from build123d import *

# Parameters (mm, degrees)
SKETCH1_R           = 4.05
BOSS_EXTRUDE1_DEPTH = 40
SKETCH2_R           = 2.75
CUT_EXTRUDE1_DEPTH  = 40
CHAMFER1_SIZE       = 5
SKETCH4_W           = 15
SKETCH4_H           = 40
BOSS_EXTRUDE2_DEPTH = 20
SKETCH5_R           = 2.75
BOSS_EXTRUDE3_DEPTH = 3
CHAMFER2_SIZE       = 5
CHAMFER3_SIZE       = 5
BOSS_EXTRUDE4_START = -5
SKETCH6_R           = 4.05
BOSS_EXTRUDE4_DEPTH = 5
SKETCH7_R           = 1.95
CUT_EXTRUDE2_DEPTH  = 20
CHAMFER4_SIZE       = 2
CHAMFER5_SIZE       = 3
SKETCH8_R           = 3
SKETCH8_R_2         = 2.75
BOSS_EXTRUDE5_DEPTH = 0.5
CHAMFER6_SIZE       = 0.5
BOSS_EXTRUDE6_START = 0.5
SKETCH9_R           = 3
SKETCH9_R_2         = 2.75
BOSS_EXTRUDE6_DEPTH = 0.5
CHAMFER7_SIZE       = 0.5


with BuildPart() as part:
    # Sketch1 → Boss-Extrude1 (new body)
    with BuildSketch(Plane.XY):
        Polygon((-20.25, 0), (20.25, 0), (20.25, -27), (41.75, -27), (41.75, 7), (-41.75, 7), (-41.75, -27), (-20.25, -27), align=None)
        with Locations((31.75, -10)):
            Circle(SKETCH1_R, mode=Mode.SUBTRACT)
        with Locations(Location((-31.75, -10, 0), (0, 0, 180))):
            Circle(SKETCH1_R, mode=Mode.SUBTRACT)
    extrude(amount=BOSS_EXTRUDE1_DEPTH)

    # Sketch2 → Cut-Extrude1 (cut)
    with BuildSketch(Plane(origin=(0, 0, 0), x_dir=(-1, 0, 0), z_dir=(0, -1, 0))):
        with Locations(Location((0, -30, 0), (0, 0, 90))):
            Circle(SKETCH2_R)
    extrude(amount=-CUT_EXTRUDE1_DEPTH, mode=Mode.SUBTRACT)

    # Chamfer1
    chamfer1_edges = [part.edges().sort_by_distance(p)[0] for p in [
        (41.75, 7, 20),
    ]]
    chamfer(chamfer1_edges, length=CHAMFER1_SIZE)

    # Sketch4 → Boss-Extrude2 (add)
    with BuildSketch(Plane(origin=(0, 7, 0), x_dir=(1, 0, 0), z_dir=(0, 1, 0))):
        with Locations((29.25, -20)):
            Rectangle(SKETCH4_W, SKETCH4_H)
    extrude(amount=BOSS_EXTRUDE2_DEPTH)

    # Sketch5 → Boss-Extrude3 (add)
    with BuildSketch(Plane(origin=(0, 27, 0), x_dir=(1, 0, 0), z_dir=(0, 1, 0))):
        with BuildLine():
            Line((20.579588566, -40), (21.75, -40))
            Line((21.75, -40), (36.75, -40))
            Line((36.75, -40), (36.75, 0))
            Line((36.75, 0), (21.75, 0))
            Line((21.75, 0), (-4.223300645, -25.738107033))
            ThreePointArc((-4.223300645, -25.738107033), (-5.538041345, -27.691299485), (-6, -30))
            Line((-6, -30), (-6, -40))
            Line((-6, -40), (20.579588566, -40))
        make_face()
        with Locations(Location((0, -30, 0), (0, 0, 90))):
            Circle(SKETCH5_R, mode=Mode.SUBTRACT)
    extrude(amount=BOSS_EXTRUDE3_DEPTH)

    # Chamfer2
    chamfer2_edges = [part.edges().sort_by_distance(p)[0] for p in [
        (36.75, 30, 20),
    ]]
    chamfer(chamfer2_edges, length=CHAMFER2_SIZE)

    # Chamfer3
    chamfer3_edges = [part.edges().sort_by_distance(p)[0] for p in [
        (-41.75, 7, 20),
    ]]
    chamfer(chamfer3_edges, length=CHAMFER3_SIZE)

    # Sketch6 → Boss-Extrude4 (add)
    with BuildSketch(Plane.XY.offset(40).offset(BOSS_EXTRUDE4_START)):
        with Locations(Location((-31.75, -10, 0), (0, 0, 180))):
            Circle(SKETCH6_R)
        with Locations((31.75, -10)):
            Circle(SKETCH6_R)
    extrude(amount=BOSS_EXTRUDE4_DEPTH)

    # Sketch7 → Cut-Extrude2 (cut)
    with BuildSketch(Plane(origin=(0, -27, 0), x_dir=(-1, 0, 0), z_dir=(0, -1, 0))):
        with Locations(Location((-31, -5, 0), (0, 0, 90))):
            Circle(SKETCH7_R)
        with Locations(Location((-31, -25, 0), (0, 0, 90))):
            Circle(SKETCH7_R)
    cut_extrude2 = extrude(amount=-CUT_EXTRUDE2_DEPTH, mode=Mode.SUBTRACT)

    # Mirror1: Cut-Extrude2 across plane
    add(cut_extrude2.mirror(Plane(origin=(0, 0, 0), x_dir=(0, 0, 1), z_dir=(1, 0, 0))), mode=Mode.SUBTRACT)

    # Chamfer4
    chamfer4_edges = [part.edges().sort_by_distance(p)[0] for p in [
        (-6, 28.5, 40),
    ]]
    chamfer(chamfer4_edges, length=CHAMFER4_SIZE)

    # Chamfer5
    chamfer5_edges = [part.edges().sort_by_distance(p)[0] for p in [
        (21.75, 7, 20),
        (21.75, 27, 20),
    ]]
    chamfer(chamfer5_edges, length=CHAMFER5_SIZE)

    # Sketch8 → Boss-Extrude5 (add)
    with BuildSketch(Plane(origin=(0, 7, 0), x_dir=(1, 0, 0), z_dir=(0, 1, 0))):
        with Locations(Location((0, -30, 0), (0, 0, 90))):
            Circle(SKETCH8_R)
        with Locations(Location((0, -30, 0), (0, 0, 90))):
            Circle(SKETCH8_R_2, mode=Mode.SUBTRACT)
    extrude(amount=BOSS_EXTRUDE5_DEPTH)

    # Chamfer6
    chamfer6_edges = [part.edges().sort_by_distance(p)[0] for p in [
        (0, 7, 33),
    ]]
    chamfer(chamfer6_edges, length=CHAMFER6_SIZE - 0.0001)  # a hair under: the kernel refuses the full size

    # Sketch9 → Boss-Extrude6 (add)
    with BuildSketch(Plane(origin=(0, 27, 0), x_dir=(-1, 0, 0), z_dir=(0, -1, 0)).offset(BOSS_EXTRUDE6_START)):
        with Locations(Location((0, -30, 0), (0, 0, 270))):
            Circle(SKETCH9_R)
        with Locations(Location((0, -30, 0), (0, 0, 90))):
            Circle(SKETCH9_R_2, mode=Mode.SUBTRACT)
    extrude(amount=-BOSS_EXTRUDE6_DEPTH)

    # Chamfer7
    chamfer7_edges = [part.edges().sort_by_distance(p)[0] for p in [
        (0, 27, 27),
    ]]
    chamfer(chamfer7_edges, length=CHAMFER7_SIZE - 0.0001)  # a hair under: the kernel refuses the full size


solid = part.part
Here's how the part is built. I have some questions about the finished solid (model axes, mm). A direction names the side the tool comes from. Give positions to 0.01 mm unless a question says otherwise; leave off trailing zeros. Loops run counter-clockwise (first coordinate to the right, second up) from the corner with the lowest first, then second, coordinate; pieces in that order, holes last. Notation, with made-up numbers: (45, 34.25) -> (62, 34.25) arc R21 cw to (62, 50.25) -> close; hole circle Ø2 at (65, -5). An arc over 180 degrees is marked (long way). Answer as a JSON object with one key per item and string values. Group by question number.
Item 1: I need wall thicknesses on L1, parallel to X at y = -22, z = 5; L2, parallel to Z at x = -31, y = -17.75; L3, parallel to X at y = -12, z = 29. Which ranges of each line are inside material? Lowest first, please.
Item 2: Imagine slicing it at B-B on y = -23. Write out the boundary of the cut face in (x, z).
Item 3: Imagine slicing it at C-C on x = -31. Write out the boundary of the cut face in (y, z), then the cut area to 3 significant figures.
Item 4: Thinking about a two-plate mould opening in Y: for faces 1 (the flat face through (-31, -27, 20)), 2 (the cylindrical face through (33.927, -6.585, 17.255)), 3 (the flat face through (9, 27, 25)), 4 (the flat face through (-41.75, -12, 20)), which applies, pulls with the +Y half, pulls with the -Y half, needs draft (parallel to the pull), parting line crosses it, or undercut?
Item 5: Imagine slicing it at D-D on z = 14. Write out the boundary of the cut face in (x, y), then the cut area to 3 significant figures.
Item 6: On a 3-axis mill with a long thin cutter (end or side, diameter ignored), from which of +Z, -Z, +X, -X, +Y, -Y can I reach the whole of each face in a straight line? I mean faces 5 (the flat face through (36.75, 16, 20)), 6 (the flat face through (0, 0, 20)), 7 (the cylindrical face through (-29.096, -20.107, 25.423)), 8 (the flat face through (-32, -10, 35)). Say none if no direction works.
Item 7: Will these pins go through, and if not, where does the flat tip stop? pin 1 (4 mm diameter, centred on x = 31, y = -9, fed in from -Z); pin 2 (2.5 mm diameter, centred on x = -31, z = 25, fed in from +Y); pin 3 (6.5 mm diameter, centred on x = -0.5, z = 31, fed in from -Y).
Item 8: Imagine slicing it at A-A on y = -3.5. Write out the boundary of the cut face in (x, z), then the cut area to 3 significant figures.
Answer list:
{
 "1": {"L1": "x = -41.75 to -32.95, -29.05 to -20.25, 20.25 to 29.05, 32.95 to 41.75", "L2": "z = 0 to 3.05, 6.95 to 23.05, 26.95 to 40", "L3": "x = -41.75 to -35.27, -28.23 to -20.25, 20.25 to 28.23, 35.27 to 41.75"},
 "2": {"outline": "(-41.75, 0) -> (-20.25, 0) -> (-20.25, 40) -> (-41.75, 40) -> close; (20.25, 0) -> (41.75, 0) -> (41.75, 40) -> (20.25, 40) -> close; hole circle Ø3.9 at (-31, 5); hole circle Ø3.9 at (-31, 25); hole circle Ø3.9 at (31, 5); hole circle Ø3.9 at (31, 25)"},
 "3": {"outline": "(-27, 0) -> (-13.98, 0) -> (-13.98, 3.05) -> (-27, 3.05) -> close; (-27, 6.95) -> (-13.98, 6.95) -> (-13.98, 23.05) -> (-27, 23.05) -> close; (-27, 26.95) -> (-13.98, 26.95) -> (-13.98, 35) -> (-6.02, 35) -> (-6.02, 0) -> (7, 0) -> (7, 40) -> (-27, 40) -> close", "area": "980 mm2"},
 "4": {"face 1": "pulls with the -Y half", "face 2": "undercut", "face 3": "undercut", "face 4": "needs draft"},
 "5": {"outline": "(-41.75, -27) -> (-20.25, -27) -> (-20.25, 0) -> (20.25, 0) -> (20.25, -27) -> (41.75, -27) -> (41.75, 2) -> (36.75, 7) -> (36.75, 25) -> (31.75, 30) -> (7.62, 30) -> (7.62, 27) -> (18.75, 27) -> (21.75, 24) -> (21.75, 10) -> (18.75, 7) -> (-36.75, 7) -> (-41.75, 2) -> close; hole circle Ø8.1 at (-31.75, -10); hole circle Ø8.1 at (31.75, -10)", "area": "2,000 mm2"},
 "6": {"face 5": "+Z, -Z, +X, +Y", "face 6": "+Z, -Z, -Y", "face 7": "-Y", "face 8": "-Z"},
 "7": {"pin 1": "stops at z = 35", "pin 2": "stops at y = 7", "pin 3": "stops at y = 0"},
 "8": {"outline": "(-41.75, 0) -> (-20.25, 0) -> (-20.25, 40) -> (-41.75, 40) -> close; (20.25, 0) -> (41.75, 0) -> (41.75, 40) -> (20.25, 40) -> close", "area": "1,720 mm2"}
}
